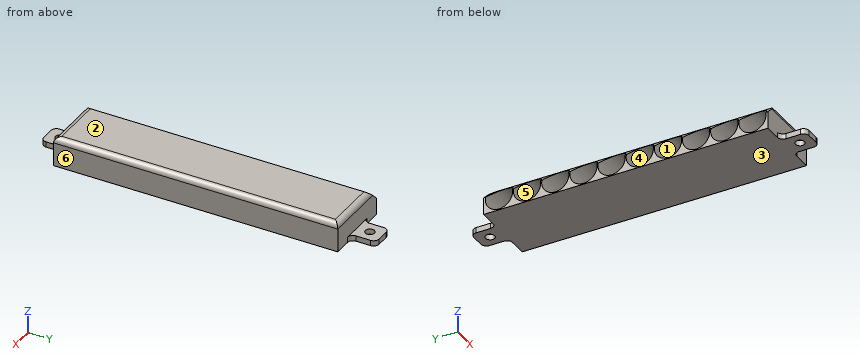
from build123d import *

# Parameters (mm, degrees)
SKETCH_1_W          = 38
SKETCH_1_H          = 16
EXTRUDE_1_DEPTH     = 156.5
SKETCH_2_R          = 7.5
CUT_EXTRUDE_1_DEPTH = 34
SKETCH_3_W          = 13
SKETCH_3_H          = 3
EXTRUDE_2_DEPTH     = 14
SKETCH_5_R          = 2.5
CUT_EXTRUDE_2_DEPTH = 3
FILLET_1_R          = 3
CUT_EXTRUDE_3_DEPTH = 156.5
MIRROR_START        = -8
MIRROR_10_OUTLINE_R = 2.5
MIRROR_10_DEPTH     = 3
FILLET_9_R          = 3
FILLET_10_R         = 3


# Read off the part's stored shape, not the designer's step: Зеркальное отражение10
with BuildPart() as part:
    # Эскиз1 → Бобышка-Вытянуть1 (new body)
    with BuildSketch(Plane(origin=(0, 0, 0), x_dir=(1, 0, 0), z_dir=(0, 1, 0))):
        Rectangle(SKETCH_1_W, SKETCH_1_H)
    extrude(amount=EXTRUDE_1_DEPTH)

    # Эскиз2 → Вырез-Вытянуть1 (cut)
    with BuildSketch(Plane.ZY.offset(19)):
        with Locations((0, 8.5)):
            Circle(SKETCH_2_R)
        with Locations((0, 24)):
            Circle(SKETCH_2_R)
        with Locations((0, 39.5)):
            Circle(SKETCH_2_R)
        with Locations((0, 55)):
            Circle(SKETCH_2_R)
        with Locations((0, 70.5)):
            Circle(SKETCH_2_R)
        with Locations((0, 86)):
            Circle(SKETCH_2_R)
        with Locations((0, 101.5)):
            Circle(SKETCH_2_R)
        with Locations((0, 117)):
            Circle(SKETCH_2_R)
        with Locations((0, 132.5)):
            Circle(SKETCH_2_R)
        with Locations((0, 148)):
            Circle(SKETCH_2_R)
    extrude(amount=-CUT_EXTRUDE_1_DEPTH, mode=Mode.SUBTRACT)

    # Эскиз3 → Бобышка-Вытянуть2 (add)
    with BuildSketch(Plane(origin=(0, 156.5, 0), x_dir=(1, 0, 0), z_dir=(0, 1, 0))):
        with Locations((-0.046570885, 6.5)):
            Rectangle(SKETCH_3_W, SKETCH_3_H)
    extrude(amount=EXTRUDE_2_DEPTH)

    # Эскиз5 → Вырез-Вытянуть2 (cut)
    with BuildSketch(Plane.XY.offset(-5)):
        with Locations((-0.023285442, 163.5)):
            Circle(SKETCH_5_R)
    extrude(amount=-CUT_EXTRUDE_2_DEPTH, mode=Mode.SUBTRACT)

    # Скругление1
    fillet_1_edges = [part.edges().sort_by_distance(p)[0] for p in [
        (-6.546570885, 156.5, -6.5),
        (6.453429115, 156.5, -6.5),
        (-6.546570885, 170.5, -6.5),
        (6.453429115, 170.5, -6.5),
    ]]
    fillet(fillet_1_edges, radius=FILLET_1_R)

    # Эскиз6 → Вырез-Вытянуть3 (cut)
    with BuildSketch(Plane.XZ):
        Polygon((-19, 1.441804302), (-12, 8), (-19, 8), align=None)
    extrude(amount=-CUT_EXTRUDE_3_DEPTH, mode=Mode.SUBTRACT)

    # Зеркальное отражение10 outline → Зеркальное отражение10 (add)
    with BuildSketch(Plane.XY.offset(MIRROR_START)):
        with BuildLine():
            Line((6.453429115, 0), (-6.546570885, 0))
            Line((-6.546570885, 0), (-6.546570885, -11))
            ThreePointArc((-6.546570885, -11), (-5.667891229, -13.121320343), (-3.546570885, -14))
            Line((-3.546570885, -14), (3.453429115, -14))
            ThreePointArc((3.453429115, -14), (5.574749459, -13.121320344), (6.453429115, -11))
            Line((6.453429115, -11), (6.453429115, 0))
        make_face()
        with Locations((-0.023285442, -7)):
            Circle(MIRROR_10_OUTLINE_R, mode=Mode.SUBTRACT)
    extrude(amount=MIRROR_10_DEPTH)

    # Скругление9
    fillet_9_edges = [part.edges().sort_by_distance(p)[0] for p in [
        (-6.546570885, 0, -6.5),
        (6.453429115, 0, -6.5),
    ]]
    fillet(fillet_9_edges, radius=FILLET_9_R)

    # Скругление10
    fillet_10_edges = [part.edges().sort_by_distance(p)[0] for p in [
        (3.5, 0, 8),
        (3.5, 156.5, 8),
        (19, 78.25, 8),
    ]]
    fillet(fillet_10_edges, radius=FILLET_10_R)


solid = part.part
Source: CAD feature listing. Evaluate the final solid. Frame: model axes, mm. Face numbers are marked on the shaded views. A direction names the side the tool comes from. Coordinates: 2 decimals unless noted, no trailing zeros. Loops run counter-clockwise (first coordinate to the right, second up) from the corner with the lowest first, then second, coordinate; pieces in that order, holes last. Notation, with made-up numbers: (29, -33.75) - (53, -33.75) arc R13 cw to (53, -29.75) - close; hole circle Ø4 at (55.5, 12.5). An arc over 180 degrees is marked (long way). One line per item, written item: value. Start each with the question number.
1. Set-up query: the marked faces 1 and 2. Return all of +Z, -Z, +X, -X, +Y, -Y with unobstructed straight access to the full face (end or side cutting, diameter ignored); none if empty.
2. Contact query for flat-ended pins moving along their axis: P1, Ø2.5, axis at y = -9, z = -6, coming from the -X side; P2, Ø0.9, axis at y = -6.5, z = -6, coming from the +X side; P3, Ø5, axis at y = 88.5, z = -1.5, coming from the -X side. Output: stop coordinate, or through.
3. Mould query, pull axis Z, two halves, no side actions, for the marked faces 3, 4, 5 and 6. Classes: pulls with the +Z half, pulls with the -Z half, needs draft (parallel to the pull), parting line crosses it, or undercut.
4. Section B-B (y = 39.5). Return the cut outline in (x, z).
5. Section C-C (y = 90.5). Return the cut outline in (x, z).
6. Ray query, L1, parallel to Z at x = -10.5, y = 24; L2, parallel to X at y = 87.5, z = 2; L3, parallel to Z at x = 12.5, y = 4. Return the intervals inside material, ascending.
7. Section A-A (x = 13). State how many separate pieces and enclosed holes the cut face has, and give its area (3 significant figures).
Verdict:
1. face 1: -X
1. face 2: +Z, +X, -X, +Y, -Y
2. P1: stops at x = -6.55
2. P2: stops at x = 6.45
2. P3: stops at x = 15
3. face 3: pulls with the -Z half
3. face 4: undercut
3. face 5: undercut
3. face 6: needs draft
4. outline: (-19, -8) - (19, -8) - (19, 5) arc R3 ccw to (16, 8) - (-12, 8) - (-12.53, 7.5) - (15, 7.5) - (15, -7.5) - (-19, -7.5) - close
5. outline: (-19, -8) - (19, -8) - (19, 5) arc R3 ccw to (16, 8) - (-12, 8) - (-14.13, 6) - (15, 6) - (15, -6) - (-19, -6) - close
6. L1: z = -8 to -7.5, 7.5 to 8
6. L2: x = 15 to 19
6. L3: z = -8 to -6, 6 to 8
7. separate pieces: 1
7. enclosed holes: 10
7. area: 733 mm2
